Geometry: see drawing. Coordinates: mm, zero at the bounding-box minimum. Give positions to 0.01 mm unless a question says otherwise; leave off trailing zeros. Write each loop counter-clockwise with the first axis right and the second up, starting at its lowest first coordinate (ties: lowest second). Pieces come first, ordered by that corner, then holes. Notation, with made-up numbers: (-33.75, -8.75) -> (-20.75, -8.75) arc R15 ccw to (-20.75, 6.25) -> close; hole circle Ø4 at (15.25, 65.5). An arc over 180 degrees is marked (long way). Write item = value, one per line.
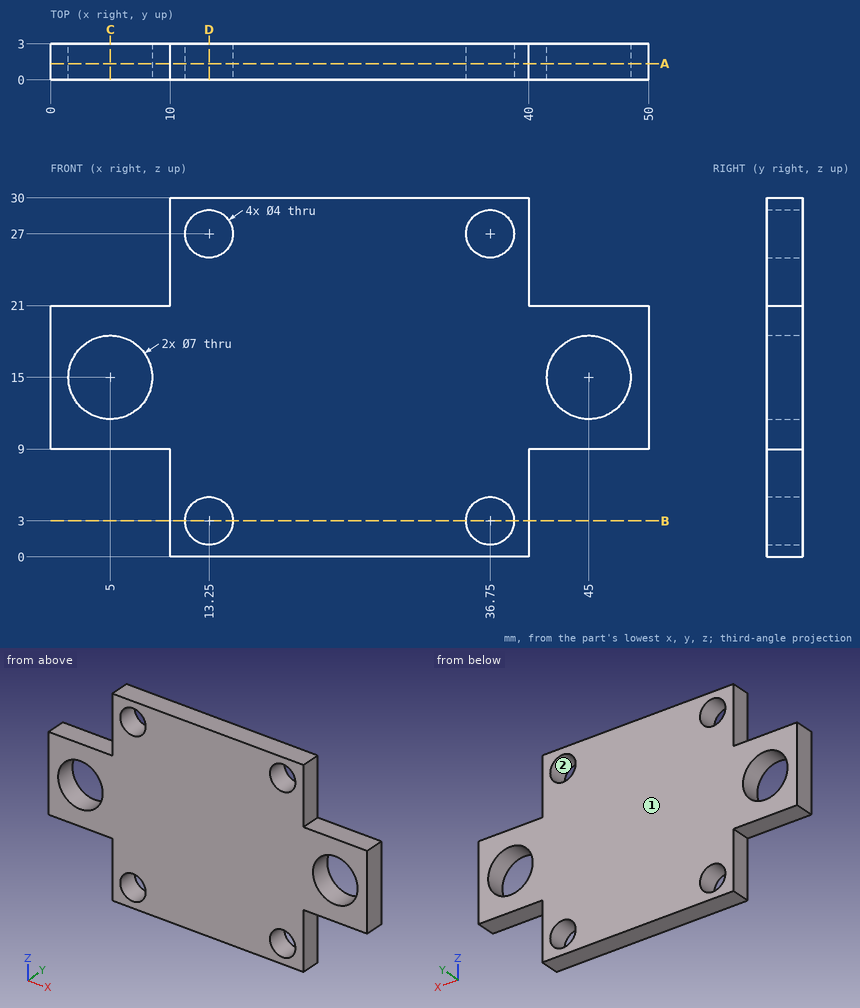
(1) Section query B-B (z = 3). Return loops of the section in (x, y), plus the area to 3 significant figures.
Values follow:
outline = (10, 0) -> (11.25, 0) -> (11.25, 3) -> (10, 3) -> close; (15.25, 0) -> (34.75, 0) -> (34.75, 3) -> (15.25, 3) -> close; (38.75, 0) -> (40, 0) -> (40, 3) -> (38.75, 3) -> close
area = 66.0 mm2
(2) Pull-direction query (Z, two-part tool) for the marked faces 1 and 2; classes: pulls with the +Z half, pulls with the -Z half, needs draft (parallel to the pull), parting line crosses it, or undercut.
Values follow:
face_1 = needs draft
face_2 = undercut
(3) Section query A-A (y = 1.35). Return loops of the section in (x, z), plus the area to 3 significant figures.
Values follow:
outline = (0, 9) -> (10, 9) -> (10, 0) -> (40, 0) -> (40, 9) -> (50, 9) -> (50, 21) -> (40, 21) -> (40, 30) -> (10, 30) -> (10, 21) -> (0, 21) -> close; hole circle Ø7 at (5, 15); hole circle Ø4 at (13.25, 3); hole circle Ø4 at (13.25, 27); hole circle Ø4 at (36.75, 3); hole circle Ø4 at (36.75, 27); hole circle Ø7 at (45, 15)
area = 1,010 mm2
(4) First-contact query: pin 1 (0.9 mm diameter, centred on x = 43.5, y = 1, fed in from -Z); pin 2 (0.9 mm diameter, centred on y = 1.5, z = 4, fed in from +X); pin 3 (0.9 mm diameter, centred on y = 1.5, z = 24, fed in from -X). Flat tips, straight axial feed; report the tip coordinate or a pass-through.
Values follow:
pin_1 = 9
pin_2 = 40
pin_3 = 10
(5) Section query D-D (x = 13.25). Return loops of the section in (y, z), plus the area to 3 significant figures.
Values follow:
outline = (0, 0) -> (3, 0) -> (3, 1) -> (0, 1) -> close; (0, 5) -> (3, 5) -> (3, 25) -> (0, 25) -> close; (0, 29) -> (3, 29) -> (3, 30) -> (0, 30) -> close
area = 66.0 mm2
(6) Section query C-C (x = 5). Return loops of the section in (y, z).
Values follow:
outline = (0, 9) -> (3, 9) -> (3, 11.5) -> (0, 11.5) -> close; (0, 18.5) -> (3, 18.5) -> (3, 21) -> (0, 21) -> close
(7) Material intervals for line 1 (X direction, y = 2.35, z = 3); line 2 (X direction, y = 2.65, z = 15.25); line 3 (Z direction, x = 11.5, y = 1.8), sorted ascending.
Values follow:
line_1 = 10 to 11.25, 15.25 to 34.75, 38.75 to 40
line_2 = 0 to 1.51, 8.49 to 41.51, 48.49 to 50
line_3 = 0 to 2.03, 3.97 to 26.03, 27.97 to 30
